Geometry check sheet. Reference: the model listing, model coordinates, mm. A direction names the side the tool comes from. Give positions to 0.01 mm unless a question says otherwise; leave off trailing zeros. Write item = value, one per line. Start each with the question number.
1. Set-up check for faces 1 (the cylindrical face through (7.83, 262.4, -93.97)), 2 (the cylindrical face through (7.83, 5.89, -6.04)), 3 (the flat face through (8, 127, -3.175)), 4 (the cylindrical face through (7.83, 252.61, -6.32)), 5 (the flat face through (8, 136, -96.838)): record each of +Z, -Z, +X, -X, +Y, -Y from which the full face is reachable in a straight line by a thin tool's end or side.
2. Thickness scan on line 1 along Y through (x, z) = (-86, -94). Record the ranges inside material, lowest first.
3. Depth check by flat-ended pin: P1, Ø5, axis at x = 7, y = 193, coming from the -Z side; P2, Ø8, axis at x = 11, y = 86.5, coming from the +Z side (3 decimals); P3, Ø8, axis at x = 11.5, z = -54.5, coming from the -Y side (3 decimals). Enter the tip coordinate at first touch or a pass-through.
```python
from build123d import *

# Parameters (mm, degrees)
BOSS_EXTRUDE1_DEPTH = 347.6625
BOSS_EXTRUDE2_DEPTH = 15.875


with BuildPart() as part:
    # Sketch1 → Boss-Extrude1 (new body)
    with BuildSketch(Plane(origin=(0, 0, 0), x_dir=(0, 0, -1), z_dir=(1, 0, 0))):
        with BuildLine():
            Line((12.7, 0), (87.3125, 0))
            ThreePointArc((87.3125, 0), (96.292756121, 3.719743879), (100.0125, 12.7))
            Line((100.0125, 12.7), (100.0125, 255.5875))
            ThreePointArc((100.0125, 255.5875), (96.292756121, 264.567756121), (87.3125, 268.2875))
            Line((87.3125, 268.2875), (12.7, 268.2875))
            ThreePointArc((12.7, 268.2875), (3.719743879, 264.567756121), (0, 255.5875))
            Line((0, 255.5875), (0, 12.7))
            ThreePointArc((0, 12.7), (3.719743879, 3.719743879), (12.7, 0))
        make_face()
    extrude(amount=-BOSS_EXTRUDE1_DEPTH)

    # Sketch2 → Boss-Extrude2 (add)
    with BuildSketch(Plane(origin=(0, 0, 0), x_dir=(0, 0, -1), z_dir=(1, 0, 0))):
        with BuildLine():
            Line((14.446389506, 256.863506359), (87.3125, 265.1125))
            ThreePointArc((87.3125, 265.1125), (94.047692091, 262.322692091), (96.8375, 255.5875))
            Line((96.8375, 255.5875), (96.8375, 12.7))
            ThreePointArc((96.8375, 12.7), (94.047692091, 5.964807909), (87.3125, 3.175))
            Line((87.3125, 3.175), (12.7, 3.175))
            ThreePointArc((12.7, 3.175), (5.964807909, 5.964807909), (3.175, 12.7))
            Line((3.175, 12.7), (3.175, 244.244113662))
            ThreePointArc((3.175, 244.244113662), (6.403111242, 252.704215515), (14.446389506, 256.863506359))
        make_face()
    extrude(amount=BOSS_EXTRUDE2_DEPTH)


solid = part.part
```
Answers:
q1.face_1 = -Z, +X, +Y
q1.face_2 = +Z, +X, -Y
q1.face_3 = +Z, +X, +Y, -Y
q1.face_4 = +Z, +X, +Y
q1.face_5 = -Z, +X, +Y, -Y
q2.line_1 = 1.9 to 266.38
q3.P1 = -96.84
q3.P2 = -3.175
q3.P3 = 3.175
